```python
from build123d import *


# Not quite as in the source:
# - a fillet or chamfer that OpenCascade refuses, or shapes differently, is made with other operations: its cross-section is extruded or revolved along the edge and cut away or added


with BuildPart() as f1:
    # F0 (on Front) → F1 (revolve)
    with BuildSketch(Plane.XZ):
        Polygon((0, 9.525), (0, 0), (406.4, 0), (406.4, 9.525), (254, 15.875), (152.4, 15.875), align=None)
    revolve(axis=Axis((203.2, 0, 0), (1, 0, 0)))

    # F2: fillet of radius 609.6 on 2 edges, made by hand

    # F2_s1 → F2_t2 (revolve, cut)
    with BuildSketch(Plane.XZ):
        with BuildLine():
            ThreePointArc((165.0944926269, 15.875), (152.4027515975, 15.7428660189), (139.7165125703, 15.3465213571))
            Line((139.7165125703, 15.3465213571), (152.4, 15.875))
            Line((152.4, 15.875), (165.0944926269, 15.875))
        make_face()
    revolve(axis=Axis((152.4, 0, 0), (1, 0, 0)), mode=Mode.SUBTRACT)

    # F2_s3 → F2_t4 (revolve, cut)
    with BuildSketch(Plane.XZ):
        with BuildLine():
            ThreePointArc((266.6834874297, 15.3465213571), (253.9972484025, 15.7428660189), (241.3055073731, 15.875))
            Line((241.3055073731, 15.875), (254, 15.875))
            Line((254, 15.875), (266.6834874297, 15.3465213571))
        make_face()
    revolve(axis=Axis((254, 0, 0), (1, 0, 0)), mode=Mode.SUBTRACT)


solid = f1.part
```
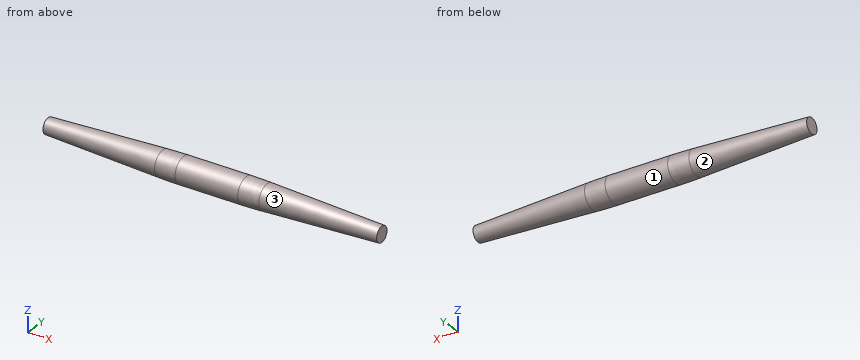
CAD build for the part. Positions are in the model's coordinates, mm. Face numbers are marked on the shaded views. Give positions to 0.01 mm unless a question says otherwise; leave off trailing zeros. Loops run counter-clockwise (first coordinate to the right, second up) from the corner with the lowest first, then second, coordinate; pieces in that order, holes last. Notation, with made-up numbers: (68.25, 68) -> (127.25, 68) arc R7 cw to (127.25, 76) -> close; hole circle Ø6 at (-38, 68). An arc over 180 degrees is marked (long way). Use a Markdown table: item, result.
1. Slice it at A-A (x = 234). List the corners of the cut face in (y, z) (3 decimals), plus the area to 3 significant figures.
Check result:
| item | result |
|---|---|
| outline | circle Ø31.75 at (0, 0) |
| area | 792 mm^2 |
2. Wall check: L1, parallel to Y at x = 191.5, z = 0.5; L2, parallel to Y at x = 138, z = -2; L3, parallel to Z at x = 122, y = -10.5. Give the ranges that are in metal, low to high. Write a range as [from, to].
Check result:
| item | result |
|---|---|
| L1 | y = [-15.87, 15.87] |
| L2 | y = [-15.14, 15.14] |
| L3 | z = [-10.16, 10.16] |
3. Slice it at B-B (x = 324). List the corners of the cut face in (y, z), plus the area to 3 significant figures.
Check result:
| item | result |
|---|---|
| outline | circle Ø25.92 at (0, 0) |
| area | 528 mm^2 |
4. Mould opens along X. For the marked faces 1, 2 and 3 say: pulls with the +X half, pulls with the -X half, needs draft (parallel to the pull), parting line crosses it, or undercut.
Check result:
| item | result |
|---|---|
| face 1 | needs draft |
| face 2 | pulls with the -X half |
| face 3 | pulls with the +X half |
5. Flat gauge pins, fed straight in: pin 1 (1 mm diameter, centred on x = 109, y = -6.5, fed in from +Z); pin 2 (3 mm diameter, centred on x = 187, y = -6.5, fed in from +Z); pin 3 (3 mm diameter, centred on x = 49, z = 8.5, fed in from -Y). Where does each tip first touch, or does it go through?
Check result:
| item | result |
|---|---|
| pin 1 | stops at z = 12.72 |
| pin 2 | stops at z = 15.07 |
| pin 3 | stops at y = -9.21 |
